Build history of the part. All positions in model axes, mm. A direction names the side the tool comes from. Round coordinates to 2 decimals unless told otherwise and drop trailing zeros. Loops run counter-clockwise (first coordinate to the right, second up) from the corner with the lowest first, then second, coordinate; pieces in that order, holes last. Notation, with made-up numbers: (51.5, 36.5) -> (92.5, 36.5) arc R37 cw to (92.5, 74.5) -> close; hole circle Ø1 at (58.25, 44). An arc over 180 degrees is marked (long way). Put each result on its own line as item: value. Start each with the question number.
Item 1: Cut at D-D, the plane x = 5. List the corners of the cut face in (y, z) (3 decimals).
Item 2: Cut at C-C, the plane z = 0.75. List the corners of the cut face in (x, y) (3 decimals), plus the area to 3 significant figures.
Item 3: Tool access for faces 1 (the flat face through (5.479, 8.346, 1.226)), 2 (the flat face through (2, 7.575, 1)), 3 (the flat face through (0, 3, 1)): list every direction of +Z, -Z, +X, -X, +Y, -Y with a clear straight run to the whole face (end or side of a thin tool).
Item 4: Pull direction Y, two halves, no side cores. Call faces 4 (the flat face through (5.4, 2, 1)), 5 (the flat face through (4, 4, 1)), 6 (the cylindrical face through (-1.099, -1.115, 1.232)): +Y half, -Y half, draft (parallel to the pull), parting line (faces both ways), or undercut.
Item 5: Cut at B-B, the plane y = 4.5. List the corners of the cut face in (x, z), plus the area to 3 significant figures.
Item 6: Drill centre lines: probe 1 along X at (y, z) = (4.75, 2.2); probe 2 along Y at (x, z) = (1, 0.2) (3 decimals); probe 3 along X at (y, z) = (5.75, 1.85). Where is each one in solid material? Low to high. Write a range as [from, to].
Item 7: Flat gauge pins, fed straight in: pin 1 Ø5 at (x, y) = (1.5, 0.5) entering from +Z; pin 2 Ø0.8 at (y, z) = (3.5, 1) entering from +X; pin 3 Ø2 at (x, z) = (2.5, 1) entering from +Y (3 decimals). Where does each tip first touch, or does it go through?
Item 8: Cut at A-A, the plane x = 0.5. List the corners of the cut face in (y, z) (3 decimals).
Autodesk Inventor part; units mm, degrees
ref_plane "YZ Plane" through (0, 0, 0) normal (1, 0, 0) x (0, 1, 0)
ref_plane "XZ Plane" through (0, 0, 0) normal (0, 1, 0) x (-1, 0, 0)
ref_plane "XY Plane" through (0, 0, 0) normal (0, 0, 1) x (1, 0, 0)
sketch "Sketch1" plane through (0, 0, 0) normal (0, 0, 1) x (1, 0, 0)
  line L0 (0, 0) -> (4, 0)
  line L1 (4, 0) -> (4, 6.175)
  line L2 (4, 6.175) -> (0, 6.175)
  line L3 (0, 6.175) -> (0, 0)
  line L4 (-0.4, -1.4) -> (4.4, -1.4)
  line L5 (5.4, -0.4) -> (5.4, 7.575)
  line L6 (5.4, 7.575) -> (-0.4, 7.575)
  line L7 (-1.4, 6.575) -> (-1.4, -0.4)
  arc A0 (-0.4, 7.575) -> (-1.4, 6.575) centre (-0.4, 6.575) ccw
  arc A1 (-1.4, -0.4) -> (-0.4, -1.4) centre (-0.4, -0.4) ccw
  arc A2 (4.4, -1.4) -> (5.4, -0.4) centre (4.4, -0.4) ccw
  point P0 (-1.4, -1.4)
  point P1 (5.4, -1.4)
  point P2 (-1.4, 7.575)
  dimension "d0" = 4
  dimension "d1" = 6.175
  dimension "d2" = 1.4
  dimension "d5" = 1
extrude "Extrusion1" add sketch "Sketch1" along normal blind 2.5
sketch "草圖3" plane through (4, 6.175, 0) normal (-1, 0, 0) x (0, 0, 1)
  line L0 (0, -6.175) -> (0, 0)
  line L1 (-0.5, 2.3) -> (3, 2.3)
  line L2 (3.5, 1.8) -> (3.5, -0.4)
  line L3 (3, -0.9) -> (-0.5, -0.9)
  line L4 (-1, -0.4) -> (-1, 1.8)
  line L5 (0, -7.575) -> (2.5, -7.575)
  arc A0 (-0.5, 2.3) -> (-1, 1.8) centre (-0.5, 1.8) ccw
  arc A1 (-1, -0.4) -> (-0.5, -0.9) centre (-0.5, -0.4) ccw
  arc A2 (3, -0.9) -> (3.5, -0.4) centre (3, -0.4) ccw
  arc A3 (3.5, 1.8) -> (3, 2.3) centre (3, 1.8) ccw
  point P0 (-1, 2.3)
  point P1 (3.5, -0.9)
  point P2 (3.5, 2.3)
  dimension "d13" = 4.5
  dimension "d15" = 3.2
  dimension "d16" = 1
  dimension "d17" = 6.675
  dimension "d18" = 0.5
extrude "擠出3" add sketch "草圖3" against normal blind 3 draft -5
properties part number "fastener_04"
Reply:
1. outline: (-1.2, 0) -> (5.362, 0) -> (5.362, -0.5) arc R0.413 ccw to (5.775, -0.913) -> (7.975, -0.913) arc R0.413 ccw to (8.388, -0.5) -> (8.388, 3) arc R0.413 ccw to (7.975, 3.413) -> (5.775, 3.413) arc R0.413 ccw to (5.362, 3) -> (5.362, 2.5) -> (-1.2, 2.5) -> close
2. outline: (-1.4, -0.4) arc R1 ccw to (-0.4, -1.4) -> (4.4, -1.4) arc R1 ccw to (5.4, -0.4) -> (5.4, 5.397) -> (7, 5.537) -> (7, 8.213) -> (4, 8.475) -> (4, 7.575) -> (-0.4, 7.575) arc R1 ccw to (-1.4, 6.575) -> close; hole (0, 0) -> (4, 0) -> (4, 6.175) -> (0, 6.175) -> close
2. area: 41.4 mm^2
3. face 1: +Z, -Z, +X, +Y
3. face 2: +Z, -Z, -X, +Y
3. face 3: +Z, -Z
4. face 4: draft
4. face 5: undercut
4. face 6: -Y half
5. outline: (-1.4, 0) -> (0, 0) -> (0, 2.5) -> (-1.4, 2.5) -> close; (4, 0) -> (5.4, 0) -> (5.4, 2.5) -> (4, 2.5) -> close
5. area: 7.00 mm^2
6. probe 1: x = [-1.4, 0], [4, 5.4]
6. probe 2: y = [-1.4, 0], [6.175, 7.575]
6. probe 3: x = [-1.4, 0], [4, 7]
7. pin 1: stops at z = 2.5
7. pin 2: stops at x = 5.4
7. pin 3: stops at y = 7.575
8. outline: (-1.4, 0) -> (0, 0) -> (0, 2.5) -> (-1.4, 2.5) -> close; (6.175, 0) -> (7.575, 0) -> (7.575, 2.5) -> (6.175, 2.5) -> close
